Source: CAD feature listing. Evaluate the final solid. Frame: model axes, mm. Face numbers are marked on the shaded views. A direction names the side the tool comes from. Round coordinates to 2 decimals unless told otherwise and drop trailing zeros. Order: outer loops, then holes, each group sorted by start corner. A loop starts at its lowest first (then second) coordinate and runs counter-clockwise, first axis right, second up. Notation, with made-up numbers: M 24,-34 L 37,-34 A20 ccw 37,-7 Z; hole C 40.5,5 d9. An arc over 180 degrees is marked long. Use one line per item in the form item = value. Start each with the question number.
Q1. Pull-direction query (X, two-part tool) for the marked faces 6, 7, 8 and 9; classes: pulls with the +X half, pulls with the -X half, needs draft (parallel to the pull), parting line crosses it, or undercut.
Q2. Reachability of the marked faces 1, 2, 3, 4 and 5 from +Z, -Z, +X, -X, +Y, -Y: full face, straight path, thin tool, end or side. Return the list, or none.
Q3. Section A-A (y = -6.5). Return the cut outline in (x, z).
Q4. Section B-B (z = 3.5). Return the cut outline in (x, y), plus the area to 3 significant figures.
Q5. Contact query for flat-ended pins moving along their axis: pin 1 (4 mm diameter, centred on x = -32.5, z = -25.5, fed in from +Y); pin 2 (1 mm diameter, centred on x = 25, y = 10.5, fed in from -Z); pin 3 (5 mm diameter, centred on x = 42.5, z = -44, fed in from +Y). Output: stop coordinate, or through.
Q6. Material intervals for probe 1 along Y at (x, z) = (24, -50); probe 2 along Z at (x, y) = (-14.5, 7.5); probe 3 along Y at (x, z) = (-44, 32), sorted ascending.
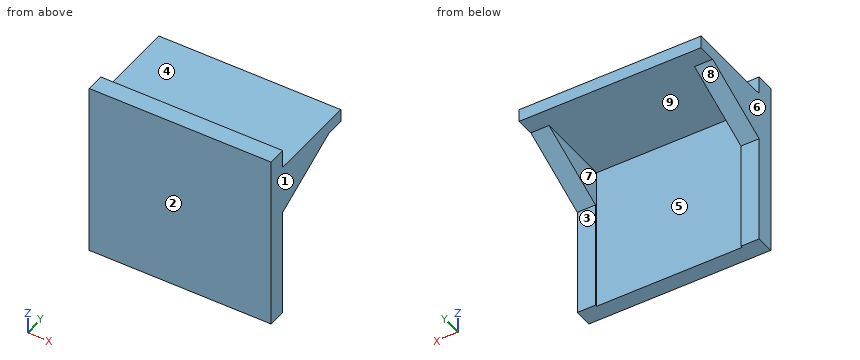
from build123d import *

# Parameters (mm, degrees)
SKETCH_1_W          = 100
SKETCH_1_H          = 60
EXTRUDE_1_DEPTH     = 37
SKETCH_2_W          = 10
SKETCH_2_H          = 50
CUT_EXTRUDE_1_DEPTH = 111.7655181
SKETCH_3_W          = 80
SKETCH_3_H          = 20
CUT_EXTRUDE_2_DEPTH = 50
CUT_EXTRUDE_3_DEPTH = 111.7655181
SKETCH_5_W          = 80
SKETCH_5_H          = 20
CUT_EXTRUDE_4_DEPTH = 1
EXTRUDE_2_DEPTH     = 60


with BuildPart() as part:
    # 草图1 → 凸台-拉伸1 (new body)
    with BuildSketch(Plane.XY):
        Rectangle(SKETCH_1_W, SKETCH_1_H)
    extrude(amount=EXTRUDE_1_DEPTH)

    # 草图2 → 切除-拉伸1 (cut, through all)
    with BuildSketch(Plane(origin=(50, 0, 0), x_dir=(0, 0, -1), z_dir=(1, 0, 0))):
        with Locations((-32, 5)):
            Rectangle(SKETCH_2_W, SKETCH_2_H)
    extrude(amount=-CUT_EXTRUDE_1_DEPTH, mode=Mode.SUBTRACT)

    # 草图3 → 切除-拉伸2 (cut)
    with BuildSketch(Plane(origin=(0, 30, 0), x_dir=(1, 0, 0), z_dir=(0, 1, 0))):
        with Locations((0, -10)):
            Rectangle(SKETCH_3_W, SKETCH_3_H)
    extrude(amount=-CUT_EXTRUDE_2_DEPTH, mode=Mode.SUBTRACT)

    # 草图4 → 切除-拉伸3 (cut, through all)
    with BuildSketch(Plane(origin=(50, 0, 0), x_dir=(0, 0, -1), z_dir=(1, 0, 0))):
        Polygon((0, 30), (-20, 30), (-20, 20), (0, -20), align=None)
    extrude(amount=-CUT_EXTRUDE_3_DEPTH, mode=Mode.SUBTRACT)

    # 草图5 → 切除-拉伸4 (cut)
    with BuildSketch(Plane(origin=(0, -20, 0), x_dir=(1, 0, 0), z_dir=(0, 1, 0))):
        with Locations((0, -10)):
            Rectangle(SKETCH_5_W, SKETCH_5_H)
    extrude(amount=-CUT_EXTRUDE_4_DEPTH, mode=Mode.SUBTRACT)

    # 草图7 → 凸台-拉伸2 (add)
    with BuildSketch(Plane(origin=(0, 0, 0), x_dir=(-1, 0, 0), z_dir=(0, 0, -1))):
        Polygon((50, -20), (40, -20), (40, -21), (-40, -21), (-40, -20), (-50, -20), (-50, -30), (50, -30), align=None)
    extrude(amount=EXTRUDE_2_DEPTH)


solid = part.part
Results list:
q1.face_6 = pulls with the -X half
q1.face_7 = undercut
q1.face_8 = needs draft
q1.face_9 = undercut
q2.face_1 = +Z, -Z, +X, +Y, -Y
q2.face_2 = +Z, -Z, +X, -X, -Y
q2.face_3 = -Z, +X, -X, +Y
q2.face_4 = +Z, +X, -X, +Y
q2.face_5 = -Z, +Y
q3.outline = M -50,6.75 L -40,6.75 L -40,20 L 40,20 L 40,6.75 L 50,6.75 L 50,27 L -50,27 Z
q4.outline = M -50,-30 L 50,-30 L 50,-13 L 40,-13 L 40,-21 L -40,-21 L -40,-13 L -50,-13 Z
q4.area = 1,060 mm2
q5.pin_1 = -21
q5.pin_2 = 20
q5.pin_3 = -20
q6.probe_1 = -30 to -21
q6.probe_2 = 20 to 27
q6.probe_3 = -30 to -20
